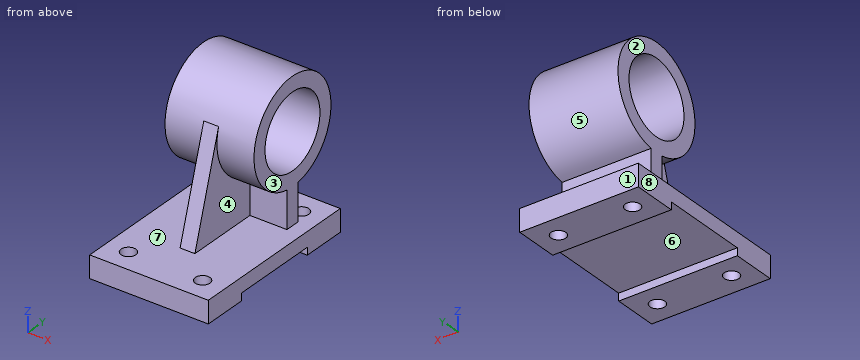
Solid Edge part; units mm, degrees
sketch "Sketch1" plane through (0, 0, 0) normal (1, 0, 0) x (0, 1, 0)
  line L0 (60, 0) -> (-60, 0)
  line L1 (-60, 0) -> (-60, -15)
  line L2 (-60, -15) -> (-30, -15)
  line L3 (-30, -15) -> (-30, -10)
  line L4 (-30, -10) -> (30, -10)
  line L5 (30, -10) -> (30, -15)
  line L6 (30, -15) -> (60, -15)
  line L7 (60, -15) -> (60, 0)
extrude "Protrusion1" add sketch "Sketch1" along normal mid plane 80
hole "Hole_1" at (-25, -45, 0) direction (0, 0, -1) diameter 10 end up to next
pattern_linear "Pattern1" count 2 spacing 50 along (1, 0, 0) count 2 spacing 90 along (0, 1, 0) of "Hole_1"
sketch "Sketch2" plane through (0, 0, 0) normal (1, 0, 0) x (0, 1, 0)
  arc A0 (25, 25) -> (35, 25) centre (30, 59.641) cw
  line L0 (35, 0) -> (35, 25)
  line L1 (35, 0) -> (25, 0)
  line L2 (25, 0) -> (25, 25)
  circle A1 centre (30, 59.641) radius 25
extrude "ExtrudedProtrusion_4" add sketch "Sketch2" along normal mid plane 60
sketch "Sketch3" plane through (0, 0, 0) normal (1, 0, 0) x (0, 1, 0)
  line L0 (-25, 0) -> (-3.4483, 69.9469)
  arc A0 (-3.4483, 69.9469) -> (25, 25) centre (30, 59.641) ccw
  line L1 (25, 0) -> (25, 25)
  line L2 (25, 0) -> (-25, 0)
extrude "ExtrudedProtrusion_3" add sketch "Sketch3" along normal mid plane 10
Design review of the part built by this model. Coordinates are the model's own, in mm. Face numbers are marked on the shaded views. A direction names the side the tool comes from. Coordinates: 2 decimals unless noted, no trailing zeros. Order: outer loops, then holes, each group sorted by start corner. A loop starts at its lowest first (then second) coordinate and runs counter-clockwise, first axis right, second up. Notation, with made-up numbers: (11.5, 13) - (34.5, 13) arc R13 ccw to (34.5, 37) - close; hole circle Ø9 at (50, 78). An arc over 180 degrees is marked (long way). One line per question, with ' | ' between items.
Q1. Consider section A-A, the plane y = -45. Give the boundary of the cut face in (x, z).
Answer key:
outline: (-40, -15) - (-30, -15) - (-30, 0) - (-40, 0) - close; (-20, -15) - (20, -15) - (20, 0) - (-20, 0) - close; (30, -15) - (40, -15) - (40, 0) - (30, 0) - close
Q2. For the marked faces 1, 2, 3, 4 and 5, list the 3-axis set-ups (+Z, -Z, +X, -X, +Y, -Y) from which the entire face can be reached by the end or side of a thin tool; tool diameter is ignored.
Answer key:
face 1: -Z, +X, -X, +Y | face 2: +Z, -X, +Y, -Y | face 3: +Z, +X, +Y, -Y | face 4: +X, -Y | face 5: none
Q3. Clearance check with flat-ended pins moving along their axes: pin 1 Ø6 at (x, y) = (-25, 45) entering from -Z; pin 2 Ø12 at (x, z) = (-1, 64.5) entering from +Y; pin 3 Ø13 at (x, y) = (25, 45) entering from +Z; pin 4 Ø13 at (x, y) = (25, -45) entering from -Z. State where each tip first meets the part, or that it passes through.
Answer key:
pin 1: stops at z = 26.76 | pin 2: stops at y = 65 | pin 3: stops at z = 93.59 | pin 4: stops at z = -15
Q4. Consider section C-C, the plane z = 37. Give the boundary of the cut face in (x, y).
Answer key:
outline: (-30, 3.31) - (-5, 3.31) - (-5, -13.6) - (5, -13.6) - (5, 3.31) - (30, 3.31) - (30, 19.4) - (-30, 19.4) - close; (-30, 40.6) - (30, 40.6) - (30, 56.69) - (-30, 56.69) - close
Q5. Consider section D-D, the plane y = 45. Give the boundary of the cut face in (x, z).
Answer key:
outline: (-40, -15) - (-30, -15) - (-30, 0) - (-40, 0) - close; (-30, 28.02) - (30, 28.02) - (30, 39.64) - (-30, 39.64) - close; (-30, 79.64) - (30, 79.64) - (30, 91.26) - (-30, 91.26) - close; (-20, -15) - (20, -15) - (20, 0) - (-20, 0) - close; (30, -15) - (40, -15) - (40, 0) - (30, 0) - close
Q6. Consider section B-B, the plane x = 21.5. Give the boundary of the cut face in (y, z), then the cut area to 3 significant figures.
Answer key:
outline: (-60, -15) - (-48.57, -15) - (-48.57, 0) - (-60, 0) - close; (-41.43, -15) - (-30, -15) - (-30, -10) - (30, -10) - (30, -15) - (41.43, -15) - (41.43, 0) - (35, 0) - (35, 25) arc R35 ccw (long way) to (25, 25) - (25, 0) - (-41.43, 0) - close; (48.57, -15) - (60, -15) - (60, 0) - (48.57, 0) - close; hole circle Ø50 at (30, 59.64) | area: 3,420 mm2
Q7. To check wall thickness, follow line 1 along Y through (x, z) = (-25, -5); line 2 along Y through (x, z) = (-25, -11); line 3 along X through (y, z) = (-45, -5). State the ranges of each line that lie inside material, in increasing order.
Answer key:
line 1: y = -60 to -50, -40 to 40, 50 to 60 | line 2: y = -60 to -50, -40 to -30, 30 to 40, 50 to 60 | line 3: x = -40 to -30, -20 to 20, 30 to 40
Q8. The part is to be moulded in two halves that separate along Z. For the marked faces 6, 7 and 8, say which applies: +Z half, -Z half, draft (parallel to the pull), parting line (faces both ways), or undercut.
Answer key:
face 6: -Z half | face 7: undercut | face 8: draft
